Input: dimensioned drawing with shaded views. Units: mm. Origin: part minimum x, y, z. Give positions to 0.01 mm unless a question says otherwise; leave off trailing zeros. Order: outer loops, then holes, each group sorted by start corner. A loop starts at its lowest first (then second) coordinate and runs counter-clockwise, first axis right, second up.
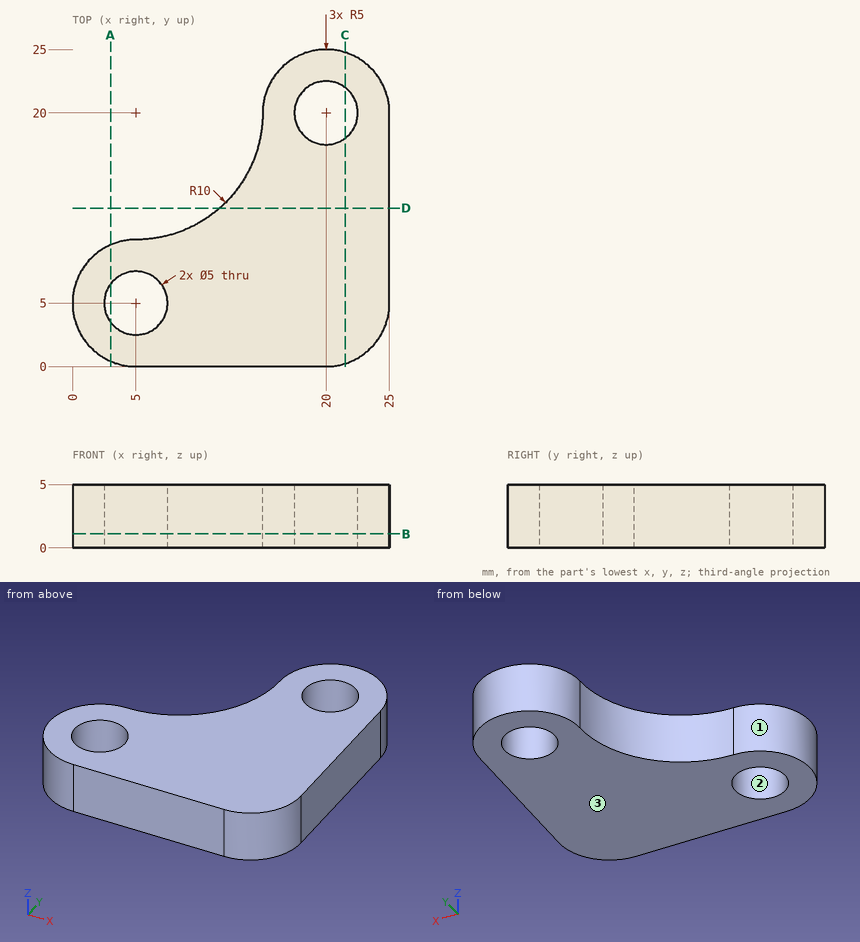
1) Section query C-C, the plane x = 21.5. Return the cut outline in (y, z), and give its area (3 significant figures).
Report:
outline: (0.23, 0) - (18, 0) - (18, 5) - (0.23, 5) - close; (22, 0) - (24.77, 0) - (24.77, 5) - (22, 5) - close
area: 103 mm2
2) Section query A-A, the plane x = 3. Return the cut outline in (y, z).
Report:
outline: (0.42, 0) - (3.5, 0) - (3.5, 5) - (0.42, 5) - close; (6.5, 0) - (9.58, 0) - (9.58, 5) - (6.5, 5) - close
3) Section query D-D, the plane y = 12.5. Return the cut outline in (x, z).
Report:
outline: (11.61, 0) - (25, 0) - (25, 5) - (11.61, 5) - close
4) Material intervals for L1, parallel to Y at x = 5, z = 1.75; L2, parallel to Y at x = 20, z = 1.3; L3, parallel to X at y = 5.75, z = 1.1, sorted ascending.
Report:
L1: y = 0 to 2.5, 7.5 to 10
L2: y = 0 to 17.5, 22.5 to 25
L3: x = 0.06 to 2.62, 7.38 to 25
5) Draft query along Y for the marked faces 1, 2 and 3. Return one class per face: +Y half, -Y half, draft (parallel to the pull), parting line (faces both ways), or undercut.
Report:
face 1: parting line
face 2: undercut
face 3: draft
6) Pin query (flat end, axial travel): pin 1 (3 mm diameter, centred on x = 10, z = 2, fed in from +Y). Return the tip coordinate at first contact, or that it passes through.
Report:
pin 1: stops at y = 12.4
7) Section query B-B, the plane z = 1.1. Return the cut outline in (x, y).
Report:
outline: (5, 0) - (20, 0) arc R5 ccw to (25, 5) - (25, 20) arc R5 ccw to (15, 20) arc R10 cw to (5, 10) arc R5 ccw to start; hole circle Ø5 at (5, 5); hole circle Ø5 at (20, 20)
